Input: part model. Units: mm. Frame: model coordinates. Face numbers are marked on the shaded views. A direction names the side the tool comes from. Coordinates: 2 decimals unless noted, no trailing zeros. Write each loop counter-clockwise with the first axis right and the second up, starting at its lowest first coordinate (ties: lowest second). Pieces come first, ordered by that corner, then holes. Notation, with made-up numbers: M -26,16.25 L -16,16.25 A16 ccw -16,31.25 Z; hole C 79,23 d10. An arc over 180 degrees is marked long. Use CSV: the item, a comma, the result in double quotes.
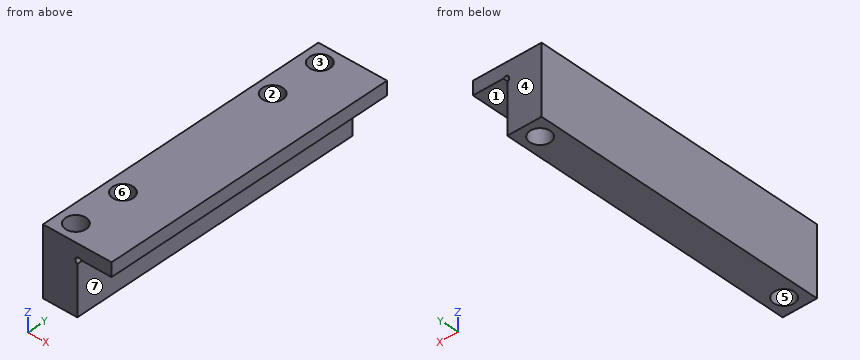
```python
from build123d import *

# Parameters (mm, degrees)
SKETCH_1_W          = 10
SKETCH_1_H          = 43.8
EXTRUDE_1_DEPTH     = 10
SKETCH_2_R          = 0.5
SKETCH_2_W          = 5
SKETCH_2_H          = 8
CUT_EXTRUDE_1_DEPTH = 57.889805765
SKETCH_3_R          = 1.5
CUT_EXTRUDE_2_DEPTH = 43.398349024
SKETCH_4_R          = 1.5
CUT_EXTRUDE_3_DEPTH = 5


with BuildPart() as part:
    # 草圖1 → 填料-伸長1 (new body)
    with BuildSketch(Plane.XY):
        with Locations((-29.9, 0)):
            Rectangle(SKETCH_1_W, SKETCH_1_H)
    extrude(amount=-EXTRUDE_1_DEPTH)

    # 草圖2 → 除料-伸長1 (cut, through all)
    with BuildSketch(Plane.XZ.offset(21.9)):
        with Locations((-29.683988881, -2.34561779)):
            Circle(SKETCH_2_R)
        with Locations((-27.4, -6)):
            Rectangle(SKETCH_2_W, SKETCH_2_H)
    extrude(amount=-CUT_EXTRUDE_1_DEPTH, mode=Mode.SUBTRACT)

    # 草圖3 → 除料-伸長2 (cut, through all)
    with BuildSketch(Plane.XY):
        with Locations((-32.4, 19.4)):
            Circle(SKETCH_3_R)
        with Locations(Location((-32.4, -19.4, 0), (0, 0, 180))):
            Circle(SKETCH_3_R)
    extrude(amount=-CUT_EXTRUDE_2_DEPTH, mode=Mode.SUBTRACT)

    # 草圖4 → 除料-伸長3 (cut)
    with BuildSketch(Plane.XY):
        with Locations((-32.4, 11.9)):
            Circle(SKETCH_4_R)
        with Locations(Location((-32.4, -11.9, 0), (0, 0, 180))):
            Circle(SKETCH_4_R)
    extrude(amount=-CUT_EXTRUDE_3_DEPTH, mode=Mode.SUBTRACT)


solid = part.part
```
1. Section D-D (y = -11.9). Return loops of the section in (x, z).
Resolved:
outline,"M -34.9,-10 L -29.9,-10 L -29.9,-2.8 A0.5 cw long -29.32,-2 L -24.9,-2 L -24.9,0 L -30.9,0 L -30.9,-5 L -33.9,-5 L -33.9,0 L -34.9,0 Z"
2. Material intervals for line 1 (Y direction, x = -32.4, z = -1.35); line 2 (Y direction, x = -32.4, z = -6); line 3 (Y direction, x = -33.25, z = -8.5), sorted ascending. Write a range as [from, to].
Resolved:
line 1,"y = [-21.9, -20.9], [-17.9, -13.4], [-10.4, 10.4], [13.4, 17.9], [20.9, 21.9]"
line 2,"y = [-21.9, -20.9], [-17.9, 17.9], [20.9, 21.9]"
line 3,"y = [-21.9, -20.64], [-18.16, 18.16], [20.64, 21.9]"
3. Section A-A (y = 19.4). Return loops of the section in (x, z), then the cut area to 3 significant figures.
Resolved:
outline,"M -34.9,-10 L -33.9,-10 L -33.9,0 L -34.9,0 Z; M -30.9,-10 L -29.9,-10 L -29.9,-2.8 A0.5 cw long -29.32,-2 L -24.9,-2 L -24.9,0 L -30.9,0 Z"
area,"29.7 mm^2"
4. Section B-B (x = -32.4). Return loops of the section in (y, z), then the cut area to 3 significant figures.
Resolved:
outline,"M -21.9,-10 L -20.9,-10 L -20.9,0 L -21.9,0 Z; M -17.9,-10 L 17.9,-10 L 17.9,0 L 13.4,0 L 13.4,-5 L 10.4,-5 L 10.4,0 L -10.4,0 L -10.4,-5 L -13.4,-5 L -13.4,0 L -17.9,0 Z; M 20.9,-10 L 21.9,-10 L 21.9,0 L 20.9,0 Z"
area,"348 mm^2"
5. Section C-C (z = -4.5). Return loops of the section in (x, y), then the cut area to 3 significant figures.
Resolved:
outline,"M -34.9,-21.9 L -29.9,-21.9 L -29.9,21.9 L -34.9,21.9 Z; hole C -32.4,-19.4 d3; hole C -32.4,-11.9 d3; hole C -32.4,11.9 d3; hole C -32.4,19.4 d3"
area,"191 mm^2"
6. Access query for the marked faces 1, 2 and 3. Directions: +Z, -Z, +X, -X, +Y, -Y. A direction counts if a zero-diameter tool reaches every point of the face in a straight line with its end or side. Return the directions, or none.
Resolved:
face 1,"-Z, +X, +Y, -Y"
face 2,"+Z"
face 3,"+Z, -Z"
7. Mould query, pull axis X, two halves, no side actions, for the marked faces 4, 5, 6 and 7. Classes: pulls with the +X half, pulls with the -X half, needs draft (parallel to the pull), parting line crosses it, or undercut.
Resolved:
face 4,"needs draft"
face 5,"undercut"
face 6,"undercut"
face 7,"pulls with the +X half"
8. Contact query for flat-ended pins moving along their axis: pin 1 Ø1.5 at (y, z) = (-1.5, -5.5) entering from +X; pin 2 Ø1.8 at (x, y) = (-32.4, -11.9) entering from +Z; pin 3 Ø3.5 at (x, y) = (-26.5, 0.5) entering from -Z. Output: stop coordinate, or through.
Resolved:
pin 1,"stops at x = -29.9"
pin 2,"stops at z = -5"
pin 3,"stops at z = -2"
